Can you work these out from the drawing? Everything is in mm from the part's minimum corner. A direction names the side the tool comes from. Coordinates: 2 decimals unless noted, no trailing zeros. Loops run counter-clockwise (first coordinate to the right, second up) from the corner with the lowest first, then second, coordinate; pieces in that order, holes last.
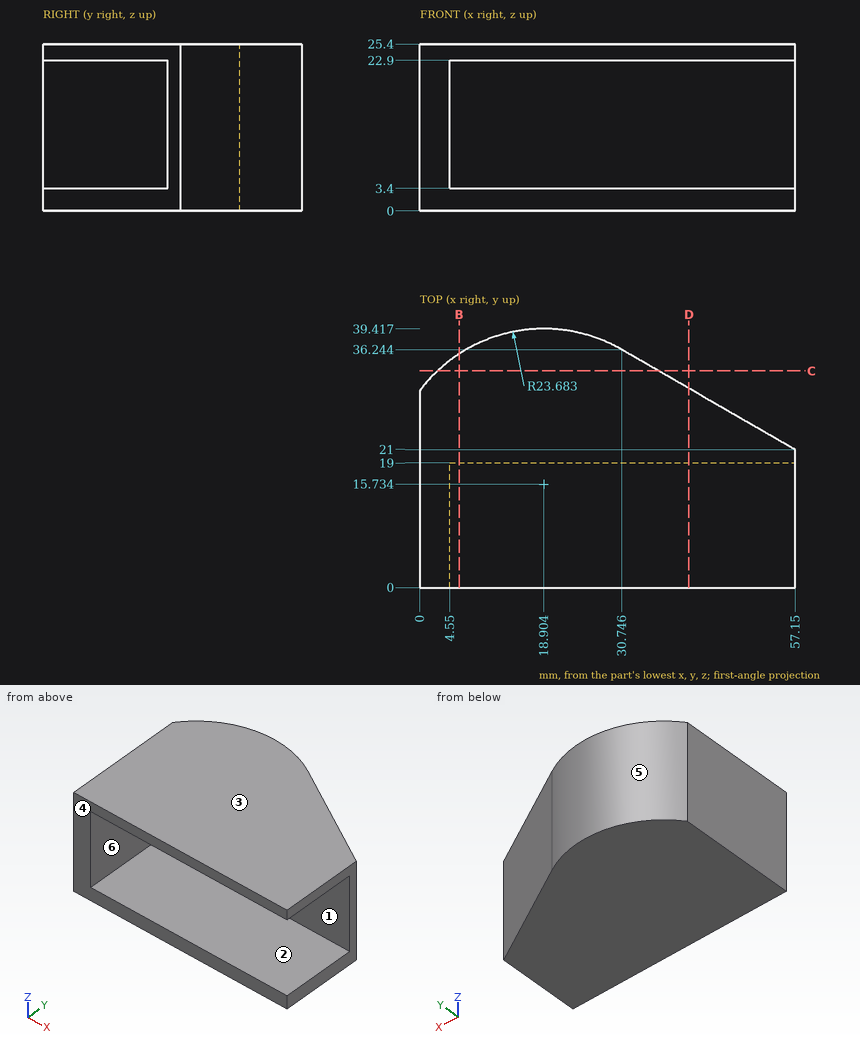
(1) We'd pull the mould along Z, two halves only. Please class the marked faces 1, 2, 3 and 4: +Z half, -Z half, draft (parallel to the pull), parting line (faces both ways), or undercut.
Answers:
face 1: undercut
face 2: undercut
face 3: +Z half
face 4: draft
(2) Imagine slicing it at C-C, the plane y = 33. Write out the boundary of the cut face in (x, z) (1 decimal), and give its area (3 significant figures).
Answers:
outline: (2.7, 0) - (36.4, 0) - (36.4, 25.4) - (2.7, 25.4) - close
area: 855 mm2
(3) For pin 1 (10 mm diameter, centred on x = 45.5, z = 12.5, fed in from +Y); pin 2 (5.5 mm diameter, centred on y = 10, z = 9, fed in from +X); pin 3 (10 mm diameter, centred on x = 26, z = 4, fed in from +Y), each with a flat end and sliding along its axis, tell me the tip position at first contact or that it passes through.
Answers:
pin 1: stops at y = 30.61
pin 2: stops at x = 4.55
pin 3: stops at y = 39.32
(4) Which directions (+Z, -Z, +X, -X, +Y, -Y) give clear straight access to the entire face, cutting with the end or side of a thin tool? Please do the marked faces 5 and 6.
Answers:
face 5: +Z, -Z, +Y
face 6: +X, -Y
(5) I need wall thicknesses on probe 1 along Z at (x, y) = (42, 13); probe 2 along X at (y, z) = (14, 21.75); probe 3 along Y at (x, z) = (53, 17.5) (1 decimal). Which ranges of each line are inside material? Lowest first, please.
Answers:
probe 1: z = 0 to 3.4, 22.9 to 25.4
probe 2: x = 0 to 4.55
probe 3: y = 19 to 23.4
(6) Imagine slicing it at D-D, the plane x = 41. Write out the boundary of the cut face in (y, z) (1 decimal), and give its area (3 significant figures).
Answers:
outline: (0, 0) - (30.3, 0) - (30.3, 25.4) - (0, 25.4) - (0, 22.9) - (19, 22.9) - (19, 3.4) - (0, 3.4) - close
area: 400 mm2
(7) Imagine slicing it at B-B, the plane x = 6. Write out the boundary of the cut face in (y, z).
Answers:
outline: (0, 0) - (35.59, 0) - (35.59, 25.4) - (0, 25.4) - (0, 22.9) - (19, 22.9) - (19, 3.4) - (0, 3.4) - close
